Geometry: final body of the model. Coordinates: model frame, mm. Give positions to 0.01 mm unless a question says otherwise; leave off trailing zeros. Loops run counter-clockwise (first coordinate to the right, second up) from the corner with the lowest first, then second, coordinate; pieces in that order, holes last. Notation, with made-up numbers: (6.25, 79.5) -> (13.25, 79.5) arc R15 cw to (13.25, 86.5) -> close; hole circle Ø10 at (-25.75, 30.5). An arc over 180 degrees is marked (long way). Answer in a Markdown table with one row per item. Add a question column.
Autodesk Inventor part; units mm, degrees
ref_plane "YZ Plane" through (0, 0, 0) normal (1, 0, 0) x (0, 1, 0)
ref_plane "XZ Plane" through (0, 0, 0) normal (0, 1, 0) x (-1, 0, 0)
ref_plane "XY Plane" through (0, 0, 0) normal (0, 0, 1) x (1, 0, 0)
sketch "Sketch1" plane through (0, 0, 0) normal (0, 0, 1) x (1, 0, 0)
  point P0 (0, 0)
sketch "Sketch2" plane through (0, 0, 0) normal (0, 0, 1) x (1, 0, 0)
  line L0 (94.9998, -95.0001) -> (-94.9998, -95.0001)
  line L1 (-94.9998, -95.0001) -> (-94.9998, 95.0001)
  line L2 (-94.9998, 95.0001) -> (94.9998, 95.0001)
  line L3 (94.9998, 95.0001) -> (94.9998, -95.0001)
  line L4 (94.9998, -95.0001) -> (-94.9998, 95.0001) construction
  line L5 (-94.9998, -95.0001) -> (94.9998, 95.0001) construction
  point P0 (0, 0)
extrude "Extrusion1" add sketch "Sketch2" along normal blind 3
sketch "Sketch3" plane through (0, 0, 3) normal (0, 0, 1) x (1, 0, 0)
  circle A0 centre (70, 80) radius 1.5001
  circle A1 centre (70, -80) radius 1.5001
  circle A2 centre (-70, 80) radius 1.5001
  circle A3 centre (-70, -80) radius 1.5001
extrude "Extrusion2" cut sketch "Sketch3" against normal blind 3
fillet "Fillet1" radius 25 1 edges at (94.9998, 95.0001, 1.5)
fillet "Fillet2" radius 25 1 edges at (94.9998, -95.0001, 1.5)
fillet "Fillet3" radius 25 1 edges at (-94.9998, -95.0001, 1.5)
fillet "Fillet4" radius 25 1 edges at (-94.9998, 95.0001, 1.5)
sketch "Pi mount holes" plane through (0, 0, 3) normal (0, 0, 1) x (1, 0, 0)
  circle A0 centre (24, -30.5) radius 1.2502
  circle A1 centre (-34, -30.5) radius 1.2502
  circle A2 centre (-34, -79.5) radius 1.2502
  circle A3 centre (24, -79.5) radius 1.2502
sketch "B205 mount holes" plane through (0, 0, 3) normal (0, 0, 1) x (1, 0, 0)
  circle A0 centre (20.32, 30.48) radius 1.5002
  circle A1 centre (-45.72, 30.48) radius 1.5002
  circle A2 centre (-45.72, -12.7) radius 1.5002
  circle A3 centre (20.32, -12.7) radius 1.5002
sketch "RM3100 mount holes" plane through (0, 0, 3) normal (0, 0, 1) x (1, 0, 0)
  circle A0 centre (0, 9) radius 0.9999
  circle A1 centre (0, -9) radius 0.9999
sketch "Pololu mount holes" plane through (0, 0, 3) normal (0, 0, 1) x (1, 0, 0)
  circle A0 centre (-73.2965, -23.9932) radius 1.1973
  circle A1 centre (-88.2965, -23.9932) radius 1.1973
  circle A2 centre (-73.2965, -59.4932) radius 1.1973
  circle A3 centre (-88.2965, -59.4932) radius 1.1973
sketch "B205 cable cutout" plane through (0, 0, 3) normal (0, 0, 1) x (1, 0, 0)
  line L0 (-76.0426, -14.5593) -> (-76.0426, 37.4411) construction
  line L1 (-81.5424, -9.0595) -> (-81.5424, 31.9413)
  line L2 (-70.5428, 31.9413) -> (-70.5428, -9.0595)
  arc A0 (-81.5424, -9.0595) -> (-70.5428, -9.0595) centre (-76.0426, -9.0595) ccw
  arc A1 (-70.5428, 31.9413) -> (-81.5424, 31.9413) centre (-76.0426, 31.9413) ccw
  point P0 (0, 0)
  point P1 (-76.0426, 11.4409)
sketch "Pi cable cutout" plane through (0, 0, 3) normal (0, 0, 1) x (1, 0, 0)
  line L0 (65.7382, -60.7056) -> (65.7382, 5.2939) construction
  line L1 (60.7378, -55.7052) -> (60.7378, 0.2935)
  line L2 (70.7387, 0.2935) -> (70.7387, -55.7052)
  arc A0 (60.7378, -55.7052) -> (70.7387, -55.7052) centre (65.7382, -55.7052) ccw
  arc A1 (70.7387, 0.2935) -> (60.7378, 0.2935) centre (65.7382, 0.2935) ccw
  point P0 (0, 0)
  point P1 (65.7382, -27.7058)
properties part number "payload_bay_square_drill_holes"
(1) Material intervals for line 1 along Y through (x, z) = (70, 1.95); line 2 along Y through (x, z) = (-69, 0.3); line 3 along X through (y, z) = (80, 0.85), sorted ascending. Write a range as from..to.
(2) Cut plane A-A on z = 2.35. Return the cut outline in (x, y).
(3) Pin query (flat end, axial travel): pin 1 Ø3.5 at (x, y) = (-70, 80) entering from -Z. Return the tip coordinate at first contact, or that it passes through.
Answer list:
| question | item | result |
|---|---|---|
| 1 | line 1 | y = -95..-81.5, -78.5..78.5, 81.5..95 |
| 1 | line 2 | y = -95..-81.12, -78.88..78.88, 81.12..95 |
| 1 | line 3 | x = -92.91..-71.5, -68.5..68.5, 71.5..92.91 |
| 2 | outline | (-95, -70) arc R25 ccw to (-70, -95) -> (70, -95) arc R25 ccw to (95, -70) -> (95, 70) arc R25 ccw to (70, 95) -> (-70, 95) arc R25 ccw to (-95, 70) -> close; hole circle Ø3 at (-70, -80); hole circle Ø3 at (-70, 80); hole circle Ø3 at (70, -80); hole circle Ø3 at (70, 80) |
| 3 | pin 1 | stops at z = 0 |
